For this review, take the finished solid that the model builds, in its own axes (mm). A direction names the side the tool comes from. Coordinates: 2 decimals unless noted, no trailing zeros. Order: outer loops, then holes, each group sorted by start corner. A loop starts at its lowest first (then second) coordinate and runs counter-clockwise, first axis right, second up. Notation, with made-up numbers: (-2, -24) -> (24, -24) arc R17 ccw to (24, -10) -> close; hole circle Ø2 at (38.5, -2). An arc over 180 degrees is marked (long way). Return JSON: item names as keys, results as strings. Group by question number.
Item 1: Draft analysis for pull direction Z (two halves, no side actions). For faces 3 (the cylindrical face through (-59.12, -6.7, 7.76)), 4 (the flat face through (48.3, -13.208, -26.2)), 5 (the cylindrical face through (-38.59, -3.13, -37.03)), 6 (the flat face through (48.2, -6.35, -11.9)), state which applies: +Z half, -Z half, draft (parallel to the pull), parting line (faces both ways), or undercut.
Item 2: Take a section at B-B (z = 0). Write out the cut boundary in (x, y), then the cut area to 3 significant figures.
Item 3: Machinability: for faces 1 (the cylindrical face through (37.03, -3.13, -38.59)), 2 (the cylindrical face through (-16.38, -9.73, -52.03)), which of the approach directions +Z, -Z, +X, -X, +Y, -Y give a long, thin tool a straight path to every point of the face, cutting with its end or side? Answer none if there is none.
Item 4: Insertion check: pin 1 (1 mm diameter, centred on x = 42.5, y = -1.5, fed in from +Z); pin 2 (4 mm diameter, centred on x = -10.5, z = -47.5, fed in from -Y); pin 3 (1 mm diameter, centred on y = -3, z = 12, fed in from +X). Each pin has a flat end and moves straight along its axis. Give the tip position at first contact, or say it passes through.
Item 5: Take a section at C-C (y = -1.75). Count the separate pieces of the cut face and the enclosed holes in it, then the cut area to 3 significant figures.
Item 6: For line 1 along X through (y, z) = (-5, -41); line 2 along Z through (x, y) = (-8.5, -5.5); line 3 along X through (y, z) = (-8.25, -23.5), list the stretches that pass through material, from the lowest coordinate up.
Item 7: Take a section at A-A (x = 0). Write out the cut boundary in (y, z), then the cut area to 3 significant figures.
Item 8: Take a section at D-D (x = 15). Write out the cut boundary in (y, z), then the cut area to 3 significant figures.
```python
from build123d import *

# Parameters (mm, degrees)
CIRPATTERN1_COUNT = 16


with BuildPart() as part:
    # Sketch1 → Revolve1 (revolve)
    with BuildSketch(Plane.XY, mode=Mode.PRIVATE) as revolve1_sk:
        Polygon((-49.4665, 0), (-59.6265, 0), (-59.6265, -13.208), (-54.5465, -13.208), (-54.5465, -6.35), (-49.4665, -6.35), align=None)
    revolve(revolve1_sk.sketch.rotate(Axis((0, 0, 0), (0, 1, 0)), 270), axis=Axis((0, 0, 0), (0, 1, 0)))

    # Sketch3 → #4 Clearance Hole1 (revolve, cut)
    with BuildSketch(Plane(origin=(0, 0, -52.26812), x_dir=(0, 0, 1), z_dir=(1, 0, 0))):
        Polygon((0, 0), (0, 11.140574487), (1.63195, 10.16), (1.63195, 0), align=None)
    f_4_clearance_hole1 = revolve(axis=Axis((0, 6.35, -52.26812), (0, -1, 0)), mode=Mode.SUBTRACT)

    # CirPattern1: #4 Clearance Hole1 ×16 about axis
    cirpattern1_axis = Axis((0, 0, 0), (0, 1, 0))
    for i in range(1, CIRPATTERN1_COUNT):
        add(f_4_clearance_hole1.rotate(cirpattern1_axis, i * 360 / CIRPATTERN1_COUNT), mode=Mode.SUBTRACT)


solid = part.part
```
Findings below:
{
 "1": {"face 3": "parting line", "face 4": "draft", "face 5": "undercut", "face 6": "undercut"},
 "2": {"outline": "(-59.63, -13.21) -> (-54.55, -13.21) -> (-54.55, -6.35) -> (-53.9, -6.35) -> (-53.9, 0) -> (-59.63, 0) -> close; (-50.64, -6.35) -> (-49.47, -6.35) -> (-49.47, 0) -> (-50.64, 0) -> close; (49.47, -6.35) -> (50.64, -6.35) -> (50.64, 0) -> (49.47, 0) -> close; (53.9, -6.35) -> (54.55, -6.35) -> (54.55, -13.21) -> (59.63, -13.21) -> (59.63, 0) -> (53.9, 0) -> close", "area": "157 mm2"},
 "3": {"face 1": "+Y, -Y", "face 2": "-Y"},
 "4": {"pin 1": "stops at z = 42.32", "pin 2": "stops at y = -6.35", "pin 3": "stops at x = 58.51"},
 "5": {"separate pieces": "1", "enclosed holes": "17", "area": "3,350 mm2"},
 "6": {"line 1": "x = -43.29 to -27.68, 27.68 to 43.29", "line 2": "z = -59.02 to -48.73, 48.73 to 59.02", "line 3": "x = -54.8 to -49.22, 49.22 to 54.8"},
 "7": {"outline": "(-13.21, -59.63) -> (0, -59.63) -> (0, -53.9) -> (-6.35, -53.9) -> (-6.35, -54.55) -> (-13.21, -54.55) -> close; (-13.21, 54.55) -> (-6.35, 54.55) -> (-6.35, 53.9) -> (0, 53.9) -> (0, 59.63) -> (-13.21, 59.63) -> close; (-6.35, -50.64) -> (0, -50.64) -> (0, -49.47) -> (-6.35, -49.47) -> close; (-6.35, 49.47) -> (0, 49.47) -> (0, 50.64) -> (-6.35, 50.64) -> close", "area": "157 mm2"},
 "8": {"outline": "(-13.21, -57.71) -> (0, -57.71) -> (0, -47.14) -> (-6.35, -47.14) -> (-6.35, -52.44) -> (-13.21, -52.44) -> close; (-13.21, 52.44) -> (-6.35, 52.44) -> (-6.35, 47.14) -> (0, 47.14) -> (0, 57.71) -> (-13.21, 57.71) -> close", "area": "206 mm2"}
}
